from build123d import *

# Parameters (mm, degrees)
BOSS_EXTRUDE2_DEPTH = 2.4
BOSS_EXTRUDE3_DEPTH = 3
SKETCH4_W           = 52
SKETCH4_H           = 2
CUT_EXTRUDE1_DEPTH  = 2.4


with BuildPart() as part:
    # Sketch1 → Boss-Extrude2 (new body)
    with BuildSketch(Plane.XY):
        Polygon((-26, -11), (36, -11), (36, -6), (26, -6), (26, -4.6), (23, -4.6), (23, -1), (26, -1), (26, 1), (23, 1), (23, 4.6), (26, 4.6), (26, 6), (36, 6), (36, 11), (-26, 11), (-26, 4.6), (-23, 4.6), (-23, 1), (-26, 1), (-26, -1), (-23, -1), (-23, -4.6), (-26, -4.6), align=None)
    extrude(amount=BOSS_EXTRUDE2_DEPTH)

    # Sketch3 → Boss-Extrude3 (add)
    with BuildSketch(Plane.XY.offset(2.4)):
        Polygon((-29.3, -14.3), (-29.3, -31.3), (-14.3, -31.3), (2.7, -14.3), (34.3, -14.3), (34.3, -31.3), (39.3, -31.3), (39.3, -14.3), (39.3, -2.7), (29.3, -2.7), (29.3, 2.7), (39.3, 2.7), (39.3, 14.3), (29.3, 14.3), (-29.3, 14.3), align=None)
    extrude(amount=BOSS_EXTRUDE3_DEPTH)

    # Sketch4 → Cut-Extrude1 (cut)
    with BuildSketch(Plane(origin=(0, 0, 0), x_dir=(-1, 0, 0), z_dir=(0, 0, -1))):
        Rectangle(SKETCH4_W, SKETCH4_H)
    extrude(amount=-CUT_EXTRUDE1_DEPTH, mode=Mode.SUBTRACT)


solid = part.part
The model under review builds one solid part; all positions refer to its coordinate system, in mm. A direction names the side the tool comes from. Give positions to 0.01 mm unless a question says otherwise; leave off trailing zeros. Order: outer loops, then holes, each group sorted by start corner. A loop starts at its lowest first (then second) coordinate and runs counter-clockwise, first axis right, second up. Notation, with made-up numbers: M -4.5,9.25 L 45.5,9.25 A24 cw 45.5,20.25 Z; hole C 64.25,88.25 d4. An arc over 180 degrees is marked long. Answer in a Markdown table with one row per item. Add a question column.
1. Add section B-B on y = -26. State the section outline as (x, z) points, plus the area to 3 significant figures.
2. Add section D-D on x = 19.5. State the section outline as (y, z) points.
3. Machinability: for faces 1 (the flat face through (29.3, 0, 4)), 2 (the flat face through (-6, -23, 4)), 3 (the flat face through (-23, 3, 1)), 4 (the flat face through (24, 4.6, 1)), which of the approach directions +Z, -Z, +X, -X, +Y, -Y give a long, thin tool a straight path to every point of the face, cutting with its end or side? Answer none if there is none.
4. Add section A-A on z = 0.8. State the section outline as (x, y) points, plus the area to 3 significant figures.
5. Mouldability with a two-part tool opening along Y and no side actions: class faces 5 (the flat face through (34, 2.7, 4)), 6 (the flat face through (31, 6, 1)), 7 (the flat face through (-29.3, -8, 4)), 8 (the flat face through (5, 11, 1)) as released by +Y, released by -Y, zero draft, split by the parting line, or undercut.
6. For pin 1 Ø0.7 at (x, z) = (5.5, 1) entering from +Y; pin 2 Ø2.5 at (y, z) = (7.5, 2) entering from +X; pin 3 Ø1.9 at (y, z) = (-3, 0.5) entering from +X; pin 4 Ø1.9 at (x, z) = (-24.5, 0.5) entering from -Y, all flat-tipped, find the tip position at first contact; note any pin that passes through.
7. To check wall thickness, follow line 1 along Y through (x, z) = (32, 3.1); line 2 along Y through (x, z) = (34.5, 4.9); line 3 along Z through (x, y) = (-16, -14). State the ranges of each line that lie inside material, in increasing order.
8. Add section C-C on x = 32. State the section outline as (y, z) points.
The answers:
| question | item | result |
|---|---|---|
| 1 | outline | M -29.3,2.4 L -9,2.4 L -9,5.4 L -29.3,5.4 Z; M 34.3,2.4 L 39.3,2.4 L 39.3,5.4 L 34.3,5.4 Z |
| 1 | area | 75.9 mm2 |
| 2 | outline | M -14.3,2.4 L -11,2.4 L -11,0 L -1,0 L -1,2.4 L 1,2.4 L 1,0 L 11,0 L 11,2.4 L 14.3,2.4 L 14.3,5.4 L -14.3,5.4 Z |
| 3 | face 1 | +Z, -Z, +X |
| 3 | face 2 | +Z, -Z, -Y |
| 3 | face 3 | -Z, -X |
| 3 | face 4 | -Z, +X |
| 4 | outline | M -26,-11 L 36,-11 L 36,-6 L 26,-6 L 26,-4.6 L 23,-4.6 L 23,-1 L -23,-1 L -23,-4.6 L -26,-4.6 Z; M -26,4.6 L -23,4.6 L -23,1 L 23,1 L 23,4.6 L 26,4.6 L 26,6 L 36,6 L 36,11 L -26,11 Z |
| 4 | area | 1,100 mm2 |
| 5 | face 5 | undercut |
| 5 | face 6 | undercut |
| 5 | face 7 | zero draft |
| 5 | face 8 | released by +Y |
| 6 | pin 1 | y = 11 |
| 6 | pin 2 | x = 39.3 |
| 6 | pin 3 | x = 23 |
| 6 | pin 4 | y = -11 |
| 7 | line 1 | -14.3 to -2.7, 2.7 to 14.3 |
| 7 | line 2 | -31.3 to -2.7, 2.7 to 14.3 |
| 7 | line 3 | 2.4 to 5.4 |
| 8 | outline | M -14.3,2.4 L -11,2.4 L -11,0 L -6,0 L -6,2.4 L -2.7,2.4 L -2.7,5.4 L -14.3,5.4 Z; M 2.7,2.4 L 6,2.4 L 6,0 L 11,0 L 11,2.4 L 14.3,2.4 L 14.3,5.4 L 2.7,5.4 Z |
